```python
from build123d import *

# Parameters (mm, degrees)
SKETCH1_R               = 3
BOSS_EXTRUDE1_DEPTH     = 18.5
CUT_EXTRUDE1_DEPTH      = 19.980252896
CUT_EXTRUDE1_DEPTH_BACK = 19.980252896
SKETCH2_R               = 1.5
CUT_SWEEP1_PROFILE_R    = 0.5


with BuildPart() as part:
    # Sketch1 → Boss-Extrude1 (new, symmetric)
    with BuildSketch(Plane.YZ):
        with Locations(Location((0, 0, 0), (0, 0, 270))):
            Circle(SKETCH1_R)
    extrude(amount=BOSS_EXTRUDE1_DEPTH, both=True)

    # Sketch2 → Cut-Extrude1 (cut, two sides: drawn at the far end of the back side and taken through both)
    with BuildSketch(Plane(origin=(0, 0, 0), x_dir=(0, 1, 0), z_dir=(0, 0, 1)).offset(-CUT_EXTRUDE1_DEPTH_BACK)):
        with Locations(Location((0, -6.5, 0), (0, 0, 270))):
            Circle(SKETCH2_R)
    extrude(amount=CUT_EXTRUDE1_DEPTH + CUT_EXTRUDE1_DEPTH_BACK, mode=Mode.SUBTRACT)

    # Cut-Sweep1: sweep along a path in Sketch3
    with BuildLine(Plane(origin=(-9.5, 0, 0), x_dir=(0, -1, 0), z_dir=(-1, 0, 0))) as cut_sweep1_path:
        CenterArc((0, 0), 3, 0, 360)
    # Cut-Sweep1 profile (on start of the path) → Cut-Sweep1 (sweep, cut)
    with BuildSketch(Plane(origin=(-9.5, -3, 0), x_dir=(1, 0, 0), z_dir=(0, 0, 1))):
        Circle(CUT_SWEEP1_PROFILE_R)
    sweep(path=cut_sweep1_path.line, mode=Mode.SUBTRACT)


solid = part.part
```
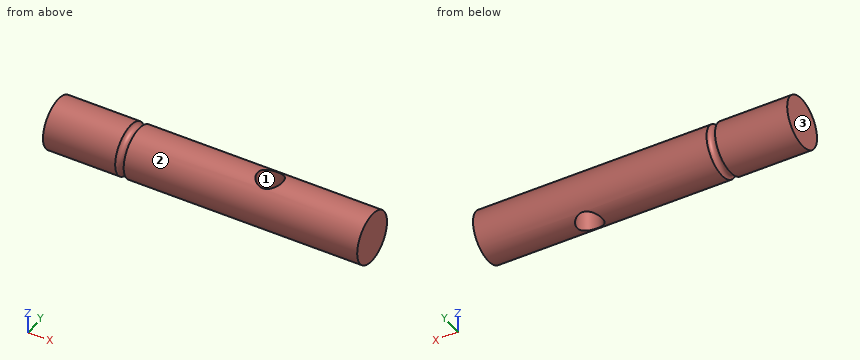
The listing builds one solid part. Answer for the finished solid, in the listing's coordinates (mm). Face numbers are marked on the shaded views. Give positions to 0.01 mm unless a question says otherwise; leave off trailing zeros. Order: outer loops, then holes, each group sorted by start corner. A loop starts at its lowest first (then second) coordinate and runs counter-clockwise, first axis right, second up. Notation, with made-up numbers: (13.25, 55.5) -> (35.25, 55.5) arc R27 cw to (35.25, 94.5) -> close; hole circle Ø10 at (-31, -3). An arc over 180 degrees is marked (long way). Write each question's results on one line, items separated by ' | '.
Q1. The part is cut by section C-C, the plane x = 6.5. Give the vertices of the cut face in (y, z), and give its area (3 significant figures).
Checked values:
outline: (-1.5, -2.6) -> (-1.5, 2.6) arc R3 ccw to start; (1.5, -2.6) arc R3 ccw to (1.5, 2.6) -> close | area: 11.1 mm^2
Q2. The part is cut by section A-A, the plane y = 0. Give the vertices of the cut face in (x, z), and give its area (3 significant figures).
Checked values:
outline: (-18.5, -3) -> (-10, -3) arc R0.5 cw to (-9, -3) -> (5, -3) -> (5, 3) -> (-9, 3) arc R0.5 cw to (-10, 3) -> (-18.5, 3) -> close; (8, -3) -> (18.5, -3) -> (18.5, 3) -> (8, 3) -> close | area: 203 mm^2
Q3. Determine the mould class of the marked faces 1, 2 and 3 for opening direction X: pulls with the +X half, pulls with the -X half, needs draft (parallel to the pull), parting line crosses it, or undercut.
Checked values:
face 1: undercut | face 2: needs draft | face 3: pulls with the -X half
Q4. Straight lines are drawn through the part: probe 1 along X at (y, z) = (0, 0.25); probe 2 along Y at (x, z) = (6.5, 0); probe 3 along Y at (x, z) = (6.5, 1.25). For each, find the intervals that lie inside material, in ascending order. Write a range as from..to.
Checked values:
probe 1: x = -18.5..5, 8..18.5 | probe 2: y = -3..-1.5, 1.5..3 | probe 3: y = -2.73..-1.5, 1.5..2.73
Q5. The part is cut by section B-B, the plane z = 0. Give the vertices of the cut face in (x, y), and give its area (3 significant figures).
Checked values:
outline: (-18.5, -3) -> (-10, -3) arc R0.5 cw to (-9, -3) -> (18.5, -3) -> (18.5, 3) -> (-9, 3) arc R0.5 cw to (-10, 3) -> (-18.5, 3) -> close; hole circle Ø3 at (6.5, 0) | area: 214 mm^2
Q6. Each of these flat-tipped pins is pushed along its axis until it touches: P1, Ø2, axis at x = -1, z = 1.5, coming from the -Y side; P2, Ø1.8, axis at x = 6.5, y = 0, coming from the -Z side; P3, Ø2, axis at x = -14.5, z = 2, coming from the +Y side. Where does it stop, or does it pass through?
Checked values:
P1: stops at y = -2.96 | P2: passes through | P3: stops at y = 2.83
